Here's the drawing with two shaded views (mm, measured from the low corner). I have some questions. A direction names the side the tool comes from. Coordinates: 2 decimals unless noted, no trailing zeros. Write each loop counter-clockwise with the first axis right and the second up, starting at its lowest first coordinate (ties: lowest second). Pieces come first, ordered by that corner, then holes. Notation, with made-up numbers: M -39.75,51.25 L -3.75,51.25 A8 ccw -3.75,63.25 Z; hole C 74,19 d1. An arc over 180 degrees is marked long. Use one line per item in the form item = value. Start each with the question number.
1. Please list where these lines run through material, in increasing order: line 1 along Y through (x, z) = (6.5, 25.5); line 2 along X through (y, z) = (26.5, 5); line 3 along X through (y, z) = (8, 22.5) (1 decimal). Write a range as [from, to].
2. On a 3-axis mill with a long thin cutter (end or side, diameter ignored), from which of +Z, -Z, +X, -X, +Y, -Y can I reach the whole of each face in a straight line? I mean the marked faces 5 and 6. Say none if no direction works.
3. Thinking about a two-plate mould opening in X: for the marked faces 1, 2, 3 and 4, which applies, released by +X, released by -X, zero draft, split by the parting line, or undercut?
4. I want a section at A-A, the plane z = 6. List the corners of the cut face in (x, y) for me, plus the area to 3 significant figures.
5. I'm going to push flat-ended pins straight in: pin 1 Ø1.2 at (x, z) = (13.5, 25) entering from -Y; pin 2 Ø3 at (x, y) = (5.5, 30) entering from +Z; pin 3 Ø2 at (x, z) = (43, 14) entering from -Y. Where does each tip first touch, or does it pass through?
6. I want a section at C-C, the plane x = 6.5. List the corners of the cut face in (y, z) for me, plus the area to 3 significant figures.
7. I want a section at D-D, the plane z = 16. List the corners of the cut face in (x, y) for me, plus the area to 3 significant figures.
8. I want a section at B-B, the plane y = 12. List the corners of the cut face in (x, z) for me (1 decimal).
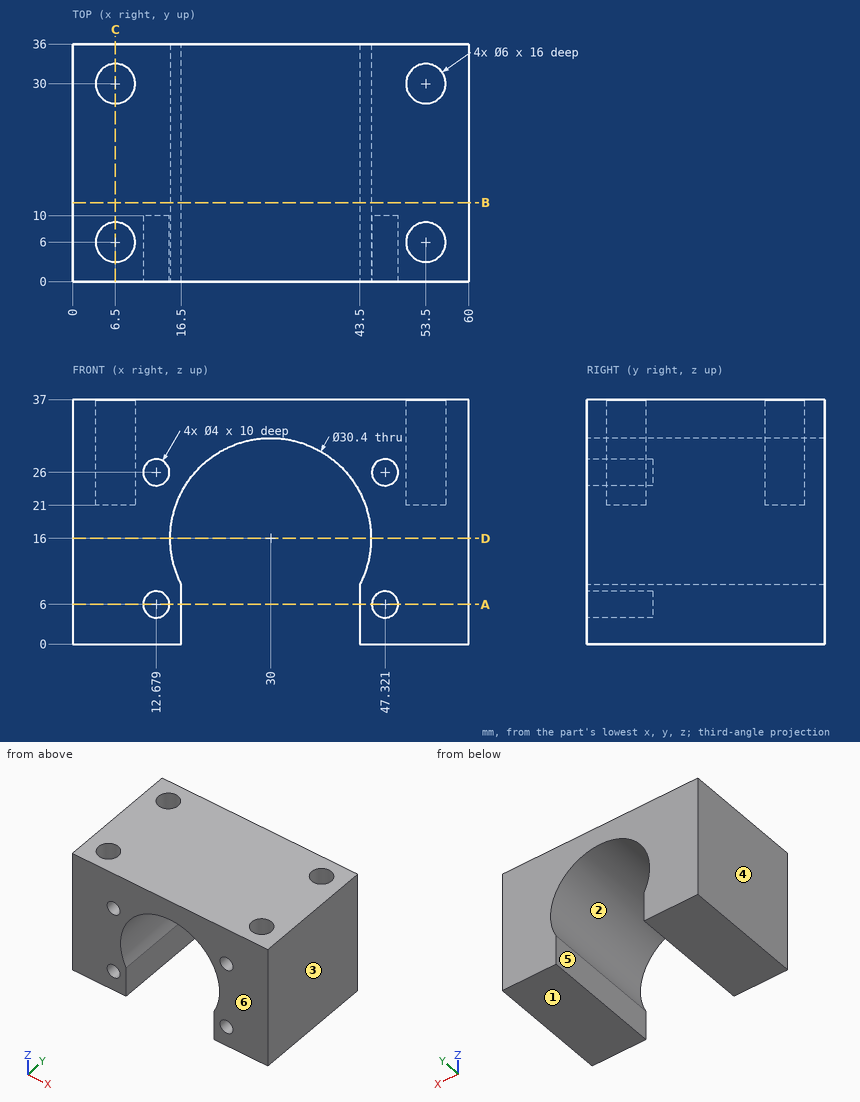
Answer list:
q1.line_1 = [0, 3], [9, 27], [33, 36]
q1.line_2 = [0, 16.5], [43.5, 60]
q1.line_3 = [0, 4.3], [8.7, 16.3], [43.7, 51.3], [55.7, 60]
q2.face_5 = -Z, +Y, -Y
q2.face_6 = +Z, -Z, +X, -X, -Y
q3.face_1 = zero draft
q3.face_2 = undercut
q3.face_3 = released by +X
q3.face_4 = released by -X
q4.outline = M 0,0 L 10.68,0 L 10.68,10 L 14.68,10 L 14.68,0 L 16.5,0 L 16.5,36 L 0,36 Z; M 43.5,0 L 45.32,0 L 45.32,10 L 49.32,10 L 49.32,0 L 60,0 L 60,36 L 43.5,36 Z
q4.area = 1,110 mm²
q5.pin_1 = 10
q5.pin_2 = 21
q5.pin_3 = through
q6.outline = M 0,0 L 36,0 L 36,37 L 33,37 L 33,21 L 27,21 L 27,37 L 9,37 L 9,21 L 3,21 L 3,37 L 0,37 Z
q6.area = 1,140 mm²
q7.outline = M 0,0 L 14.8,0 L 14.8,36 L 0,36 Z; M 45.2,0 L 60,0 L 60,36 L 45.2,36 Z
q7.area = 1,070 mm²
q8.outline = M 0,0 L 16.5,0 L 16.5,9 A15.2 cw long 43.5,9 L 43.5,0 L 60,0 L 60,37 L 0,37 Z
